```python
from build123d import *

# Parameters (mm, degrees)
CROQUIS1_W              = 170
CROQUIS1_H              = 30
CROQUIS1_W_2            = 40
CROQUIS1_H_2            = 20
SALIENTE_EXTRUIR1_DEPTH = 10
CROQUIS2_R              = 2.25
CORTAR_EXTRUIR1_DEPTH   = 10
REDONDEO3_R             = 10
CROQUIS3_R              = 1.5
CORTAR_EXTRUIR2_DEPTH   = 10


with BuildPart() as part:
    # Croquis1 → Saliente-Extruir1 (new body)
    with BuildSketch(Plane(origin=(0, 0, 0), x_dir=(1, 0, 0), z_dir=(0, 1, 0))):
        Rectangle(CROQUIS1_W, CROQUIS1_H)
        with Locations((50, 0)):
            Rectangle(CROQUIS1_W_2, CROQUIS1_H_2, mode=Mode.SUBTRACT)
    extrude(amount=SALIENTE_EXTRUIR1_DEPTH)

    # Croquis2 → Cortar-Extruir1 (cut)
    with BuildSketch(Plane(origin=(0, 10, 0), x_dir=(1, 0, 0), z_dir=(0, 1, 0))):
        with Locations(Location((74.5, -5, 0), (0, 0, 270))):
            Circle(CROQUIS2_R)
        with Locations(Location((74.5, 5, 0), (0, 0, 90))):
            Circle(CROQUIS2_R)
        with Locations(Location((25.5, -5, 0), (0, 0, 90))):
            Circle(CROQUIS2_R)
        with Locations(Location((25.5, 5, 0), (0, 0, 270))):
            Circle(CROQUIS2_R)
    extrude(amount=-CORTAR_EXTRUIR1_DEPTH, mode=Mode.SUBTRACT)

    # Redondeo3
    redondeo3_edges = [part.edges().sort_by_distance(p)[0] for p in [
        (-85, 5, -15),
        (85, 5, -15),
        (85, 5, 15),
        (-85, 5, 15),
    ]]
    fillet(redondeo3_edges, radius=REDONDEO3_R)

    # Croquis3 → Cortar-Extruir2 (cut)
    with BuildSketch(Plane(origin=(0, 10, 0), x_dir=(1, 0, 0), z_dir=(0, 1, 0))):
        with Locations(Location((-75, 0, 0), (0, 0, 270))):
            Circle(CROQUIS3_R)
    extrude(amount=-CORTAR_EXTRUIR2_DEPTH, mode=Mode.SUBTRACT)


solid = part.part
```
Check sheet for the modelled part. Datum: model origin and axes. Units: mm. A direction names the side the tool comes from. Round coordinates to 2 decimals unless told otherwise and drop trailing zeros. Loops run counter-clockwise (first coordinate to the right, second up) from the corner with the lowest first, then second, coordinate; pieces in that order, holes last. Notation, with made-up numbers: (-15, -21.5) - (26, -21.5) arc R12 cw to (26, -11.5) - close; hole circle Ø10 at (31.5, -4.75). An arc over 180 degrees is marked (long way). Write item = value, one per line. Start each with the question number.
Q1. Thickness scan on L1, parallel to X at y = 4.75, z = -5; L2, parallel to Z at x = 57.5, y = 5.75; L3, parallel to X at y = 5, z = -8. Record the ranges inside material, lowest first.
Q2. Section check B-B (x = 25.5). Record the boundary of the cut face in (y, z), plus the area to 3 significant figures.
Q3. Section check A-A (y = 6.5). Record the boundary of the cut face in (x, z), plus the area to 3 significant figures.
Q4. Depth check by flat-ended pin: P1, Ø3, axis at y = 4.5, z = 9, coming from the +X side; P2, Ø2.5, axis at x = 74.5, z = -5, coming from the +Y side; P3, Ø5, axis at x = -75, z = 0, coming from the +Y side; P4, Ø3, axis at y = 5, z = -10, coming from the +X side. Enter the tip coordinate at first touch or a pass-through.
Q5. Access from +Z, -Z, +X, -X, +Y, -Y to the whole of each face (thin tool, end or side, straight path). Record for faces 1 (the face through (30, 5, 0)), 2 (the face through (-20, 10, 0)).
Q6. Release check for a two-part mould opening along Z. For faces 3 (the face through (-85, 5, 0)), 4 (the face through (-82.15, 5.07, 11.99)), 5 (the face through (23.304, 5.07, -5.488)) record: pulls with the +Z half, pulls with the -Z half, needs draft (parallel to the pull), parting line crosses it, or undercut.
Derived:
q1.L1 = -85 to 23.25, 27.75 to 30, 70 to 72.25, 76.75 to 85
q1.L2 = -15 to -10, 10 to 15
q1.L3 = -84.54 to 30, 70 to 84.54
q2.outline = (0, -15) - (10, -15) - (10, -7.25) - (0, -7.25) - close; (0, -2.75) - (10, -2.75) - (10, 2.75) - (0, 2.75) - close; (0, 7.25) - (10, 7.25) - (10, 15) - (0, 15) - close
q2.area = 210 mm^2
q3.outline = (-85, -5) arc R10 ccw to (-75, -15) - (75, -15) arc R10 ccw to (85, -5) - (85, 5) arc R10 ccw to (75, 15) - (-75, 15) arc R10 ccw to (-85, 5) - close; hole circle Ø3 at (-75, 0); hole circle Ø4.5 at (25.5, -5); hole circle Ø4.5 at (25.5, 5); hole (30, -10) - (70, -10) - (70, 10) - (30, 10) - close; hole circle Ø4.5 at (74.5, -5); hole circle Ø4.5 at (74.5, 5)
q3.area = 4,140 mm^2
q4.P1 = 84.68
q4.P2 = through
q4.P3 = 10
q4.P4 = 84.37
q5.face_1 = +Y, -Y
q5.face_2 = +Z, -Z, +X, -X, +Y
q6.face_3 = needs draft
q6.face_4 = pulls with the +Z half
q6.face_5 = undercut
